Drawing for the job (mm, zero at the part's lowest x, y, z). A direction names the side the tool comes from. Give positions to 0.01 mm unless a question says otherwise; leave off trailing zeros. Loops run counter-clockwise (first coordinate to the right, second up) from the corner with the lowest first, then second, coordinate; pieces in that order, holes last. Notation, with made-up numbers: (-25, 24.5) -> (-12, 24.5) arc R10 cw to (-12, 31.5) -> close; hole circle Ø11 at (61, 16). An arc over 180 degrees is marked (long way). Use CSV: the item, a comma, the result in double quotes. Start each with the question number.
(1) Flat gauge pins, fed straight in: pin 1 (2 mm diameter, centred on x = 52, z = 8, fed in from -Y); pin 2 (4 mm diameter, centred on x = 21.5, z = 8.5, fed in from -Y); pin 3 (1 mm diameter, centred on x = 21, z = 7, fed in from +Y). Where does each tip first touch, or does it go through?
(2) Cut at D-D on x = 41. Write the cut outline in (y, z), then the cut area to 3 significant figures.
(3) Drill centre lines: probe 1 along X at (y, z) = (2.25, 9.5); probe 2 along Z at (x, y) = (53, 5.75); probe 3 along Y at (x, z) = (17, 6). Where is each one in solid material? Low to high.
(4) Cut at A-A on z = 6. Write the cut outline in (x, y), then the cut area to 3 significant figures.
(5) 3-axis set-ups, long thin cutter, end or side, ignore diameter. For the marked faces 1, 2 and 3: which of +Z, -Z, +X, -X, +Y, -Y reach the whole face in a straight line?
(6) Cut at C-C on x = 4.5. Write the cut outline in (y, z).
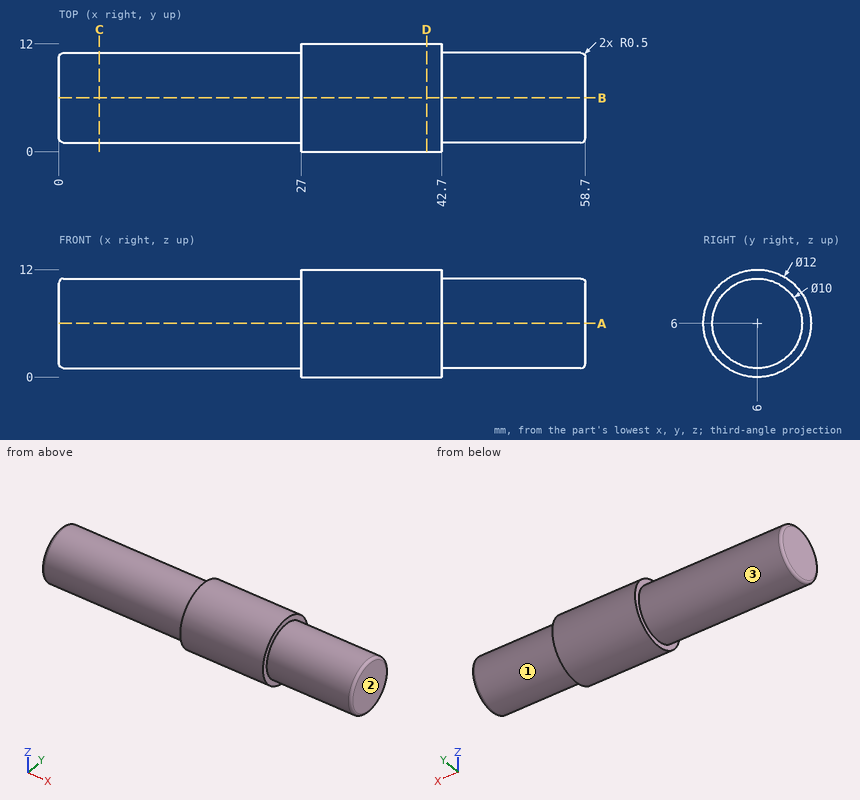
Check result:
1,pin 1,"y = 1.1"
1,pin 2,"y = 1.03"
1,pin 3,"y = 10.97"
2,outline,"circle Ø12 at (6, 6)"
2,area,"113 mm²"
3,probe 1,"27 to 42.7"
3,probe 2,"1.01 to 10.99"
3,probe 3,"1 to 11"
4,outline,"(0, 1.5) arc R0.5 ccw to (0.5, 1) -> (27, 1) -> (27, 0) -> (42.7, 0) -> (42.7, 1) -> (58.2, 1) arc R0.5 ccw to (58.7, 1.5) -> (58.7, 10.5) arc R0.5 ccw to (58.2, 11) -> (42.7, 11) -> (42.7, 12) -> (27, 12) -> (27, 11) -> (0.5, 11) arc R0.5 ccw to (0, 10.5) -> close"
4,area,"618 mm²"
5,face 1,"+X"
5,face 2,"+Z, -Z, +X, +Y, -Y"
5,face 3,"-X"
6,outline,"circle Ø10 at (6, 6)"
